Could you check a few things on this drawing? It's one solid part, dimensions in mm from its lowest x, y, z. A direction names the side the tool comes from. Give positions to 0.01 mm unless a question says otherwise; leave off trailing zeros. Write each loop counter-clockwise with the first axis right and the second up, starting at its lowest first coordinate (ties: lowest second). Pieces come first, ordered by that corner, then holes.
1. I'm going to push flat-ended pins straight in: pin 1 (1.5 mm diameter, centred on y = 3, z = 1.5, fed in from -X); pin 2 (1.5 mm diameter, centred on x = 2.5, y = 0.5, fed in from -Z). Where does each tip first touch, or does it pass through?
2. Suppose I cut it at C-C (z = 5.5). Please give me the cut outline in (x, y).
3. Suppose I cut it at A-A (z = 9). Please give me the cut outline in (x, y), and give its area (3 significant figures).
4. If I drill on probe 1 along X at (y, z) = (3.5, 8.75) (1 decimal); probe 2 along Z at (x, y) = (4.6, 4.25); probe 3 along X at (y, z) = (3.65, 6.5) (1 decimal), over which ranges is the centre line in solid material (lowest first)?
5. Thinking about a two-plate mould opening in Y: for the marked faces 3, 4 and 5, which applies, pulls with the +Y half, pulls with the -Y half, needs draft (parallel to the pull), parting line crosses it, or undercut?
6. Suppose I cut it at B-B (y = 4.8). Please give me the cut outline in (x, z), and give its area (3 significant figures).
7. On a 3-axis mill with a long thin cutter (end or side, diameter ignored), from which of +Z, -Z, +X, -X, +Y, -Y can I reach the whole of each face in a straight line? I mean the marked faces 1 and 2. Say none if no direction works.
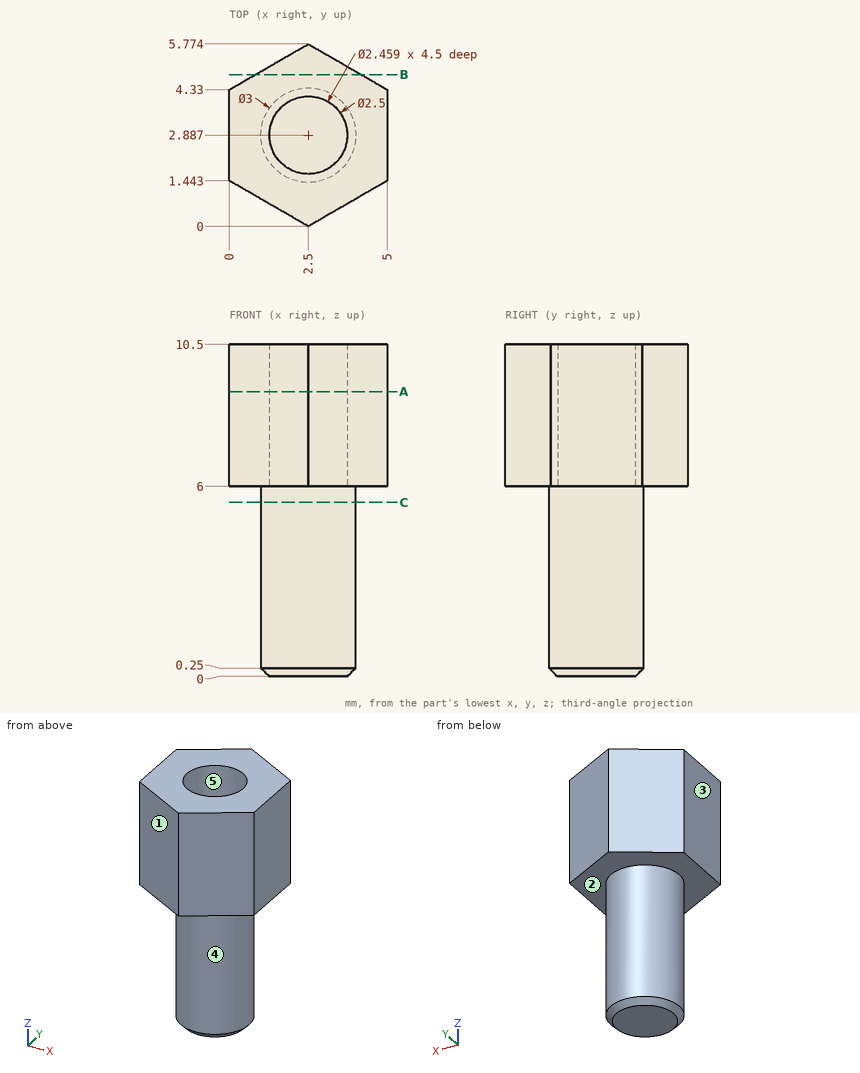
Checks:
1. pin 1: stops at x = 1
1. pin 2: stops at z = 6
2. outline: circle Ø3 at (2.5, 2.89)
3. outline: (0, 1.44) - (2.5, 0) - (5, 1.44) - (5, 4.33) - (2.5, 5.77) - (0, 4.33) - close; hole circle Ø2.46 at (2.5, 2.89)
3. area: 16.9 mm2
4. probe 1: x = 0 to 1.4, 3.6 to 5
4. probe 2: z = 6 to 10.5
4. probe 3: x = 0 to 1.5, 3.5 to 5
5. face 3: needs draft
5. face 4: parting line crosses it
5. face 5: undercut
6. outline: (0.81, 6) - (4.19, 6) - (4.19, 10.5) - (0.81, 10.5) - close
6. area: 15.2 mm2
7. face 1: +Z, -Z, -X, -Y
7. face 2: -Z
